The model under review builds one solid part; all positions refer to its coordinate system, in mm. Face numbers are marked on the shaded views. Give positions to 0.01 mm unless a question says otherwise; leave off trailing zeros. Order: outer loops, then holes, each group sorted by start corner. A loop starts at its lowest first (then second) coordinate and runs counter-clockwise, first axis right, second up.
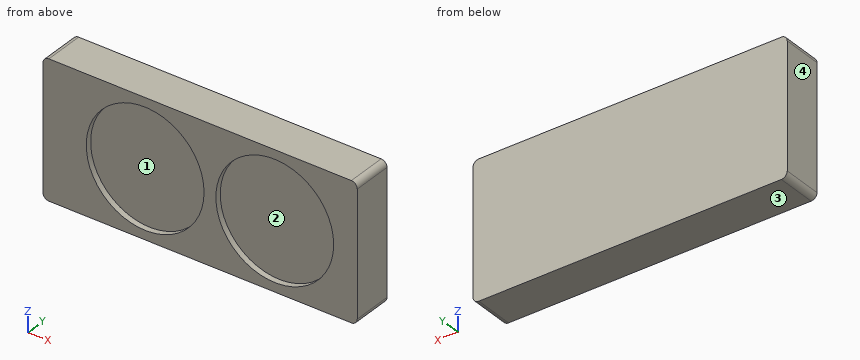
```python
from build123d import *

# Parameters (mm, degrees)
F1_DEPTH = 34
F2_R     = 50
F3_DEPTH = 5


with BuildPart() as f1:
    # F0 (on Front) → F1 (new body)
    with BuildSketch(Plane.XZ):
        with BuildLine():
            ThreePointArc((0, 5), (1.464466, 1.464466), (5, 0))
            Line((5, 0), (261.7, 0))
            ThreePointArc((261.7, 0), (265.235534, 1.464466), (266.7, 5))
            Line((266.7, 5), (266.7, 110.4))
            ThreePointArc((266.7, 110.4), (265.235534, 113.935534), (261.7, 115.4))
            Line((261.7, 115.4), (5, 115.4))
            ThreePointArc((5, 115.4), (1.464466, 113.935534), (0, 110.4))
            Line((0, 110.4), (0, 5))
        make_face()
    extrude(amount=F1_DEPTH)

    # F2 (on face) → F3 (cut)
    with BuildSketch(Plane.XZ.offset(34)):
        with Locations((86.7, 57.7)):
            Circle(F2_R)
        with Locations((196.7, 57.7)):
            Circle(F2_R)
    extrude(amount=-F3_DEPTH, mode=Mode.SUBTRACT)


solid = f1.part
```
1. To check wall thickness, follow line 1 (Z direction, x = 86.7, y = -32.4); line 2 (Y direction, x = 118, z = 60). State the ranges of each line that lie inside material, in increasing order.
2. Draft analysis for pull direction X (two halves, no side actions). For the marked faces 1, 2, 3 and 4, state which applies: pulls with the +X half, pulls with the -X half, needs draft (parallel to the pull), parting line crosses it, or undercut.
3. Insertion check: pin 1 (2 mm diameter, centred on x = 75, z = 101, fed in from -Y). The pin has a flat end and moves straight along its axis. Give the tip position at first contact, or say it passes through.
4. Take a section at C-C (z = 28.5). Write out the cut boundary in (x, y).
5. Take a section at D-D (x = 152.5). Write out the cut boundary in (y, z).
6. Take a section at B-B (z = 57.7). Write out the cut boundary in (x, y).
7. Take a section at A-A (x = 86.7). Write out the cut boundary in (y, z).
Answer:
1. line 1: z = 0 to 7.7, 107.7 to 115.4
1. line 2: y = -29 to 0
2. face 1: undercut
2. face 2: undercut
2. face 3: needs draft
2. face 4: pulls with the -X half
3. pin 1: stops at y = -29
4. outline: (0, -34) - (46.11, -34) - (46.11, -29) - (127.29, -29) - (127.29, -34) - (156.11, -34) - (156.11, -29) - (237.29, -29) - (237.29, -34) - (266.7, -34) - (266.7, 0) - (0, 0) - close
5. outline: (-34, 0) - (0, 0) - (0, 115.4) - (-34, 115.4) - (-34, 81.07) - (-29, 81.07) - (-29, 34.33) - (-34, 34.33) - close
6. outline: (0, -34) - (36.7, -34) - (36.7, -29) - (136.7, -29) - (136.7, -34) - (146.7, -34) - (146.7, -29) - (246.7, -29) - (246.7, -34) - (266.7, -34) - (266.7, 0) - (0, 0) - close
7. outline: (-34, 0) - (0, 0) - (0, 115.4) - (-34, 115.4) - (-34, 107.7) - (-29, 107.7) - (-29, 7.7) - (-34, 7.7) - close
